```python
from build123d import *

# Parameters (mm, degrees)
SKETCH1_W           = 57.15
SKETCH1_H           = 50.00625
SKETCH1_W_2         = 44.45
SKETCH1_H_2         = 37.30625
BOSS_EXTRUDE1_DEPTH = 12.7
SKETCH2_W           = 57.15
SKETCH2_H           = 50.00625
SKETCH2_R           = 6.35
BOSS_EXTRUDE2_DEPTH = 3.175
SKETCH4_W           = 12.7
SKETCH4_H           = 3.175
BOSS_EXTRUDE3_DEPTH = 12.7
SKETCH5_R           = 2.4892
CUT_EXTRUDE1_DEPTH  = 3.175
FILLET1_R           = 1.27
SKETCH6_R           = 1.5875
CUT_EXTRUDE2_DEPTH  = 9.525


with BuildPart() as part:
    # Sketch1 → Boss-Extrude1 (new body)
    with BuildSketch(Plane.XY):
        Rectangle(SKETCH1_W, SKETCH1_H)
        Rectangle(SKETCH1_W_2, SKETCH1_H_2, mode=Mode.SUBTRACT)
    extrude(amount=BOSS_EXTRUDE1_DEPTH)

    # Sketch2 → Boss-Extrude2 (add)
    with BuildSketch(Plane.XY):
        Rectangle(SKETCH2_W, SKETCH2_H)
        Circle(SKETCH2_R, mode=Mode.SUBTRACT)
    extrude(amount=-BOSS_EXTRUDE2_DEPTH)

    # Sketch4 → Boss-Extrude3 (add)
    with BuildSketch(Plane.XY):
        with Locations((-34.925, -23.415625)):
            Rectangle(SKETCH4_W, SKETCH4_H)
        with Locations((34.925, -23.415625)):
            Rectangle(SKETCH4_W, SKETCH4_H)
    extrude(amount=BOSS_EXTRUDE3_DEPTH)

    # Sketch5 → Cut-Extrude1 (cut)
    with BuildSketch(Plane(origin=(0, -21.828125, 0), x_dir=(1, 0, 0), z_dir=(0, 1, 0))):
        with Locations(Location((-34.925, -6.35, 0), (0, 0, 180))):
            Circle(SKETCH5_R)
        with Locations(Location((34.925, -6.35, 0), (0, 0, 180))):
            Circle(SKETCH5_R)
    extrude(amount=-CUT_EXTRUDE1_DEPTH, mode=Mode.SUBTRACT)

    # Fillet1
    fillet1_edges = [part.edges().sort_by_distance(p)[0] for p in [
        (-22.225, 0, 0),
        (0, -18.653125, 0),
        (22.225, 0, 0),
        (0, 18.653125, 0),
    ]]
    fillet(fillet1_edges, radius=FILLET1_R)

    # Sketch6 → Cut-Extrude2 (cut)
    with BuildSketch(Plane.XY.offset(12.7)):
        with Locations((-25.4, 21.828125)):
            Circle(SKETCH6_R)
        with Locations((25.4, 21.828125)):
            Circle(SKETCH6_R)
        with Locations((25.4, -21.828125)):
            Circle(SKETCH6_R)
        with Locations((-25.4, -21.828125)):
            Circle(SKETCH6_R)
    extrude(amount=-CUT_EXTRUDE2_DEPTH, mode=Mode.SUBTRACT)


solid = part.part
```
For this review, take the finished solid that the model builds, in its own axes (mm). A direction names the side the tool comes from. Round coordinates to 2 decimals unless told otherwise and drop trailing zeros. Write each loop counter-clockwise with the first axis right and the second up, starting at its lowest first coordinate (ties: lowest second). Pieces come first, ordered by that corner, then holes.
1) Insertion check: pin 1 Ø1 at (x, y) = (-25.5, -22.5) entering from +Z (3 decimals); pin 2 Ø1 at (x, y) = (12, 5) entering from +Z; pin 3 Ø1 at (x, y) = (-37.5, -24) entering from -Z; pin 4 Ø4.5 at (x, z) = (-34.925, 6.35) entering from +Y. Each pin has a flat end and moves straight along its axis. Give the tip position at first contact, or say it passes through.
Answer below:
pin 1: stops at z = 3.175
pin 2: stops at z = 0
pin 3: stops at z = 0
pin 4: passes through
2) Take a section at D-D on x = 0. Give the boundary of the cut face in (y, z) (3 decimals).
Answer below:
outline: (-25.003, -3.175) - (-6.35, -3.175) - (-6.35, 0) - (-17.383, 0) arc R1.27 cw to (-18.653, 1.27) - (-18.653, 12.7) - (-25.003, 12.7) - close; (6.35, -3.175) - (25.003, -3.175) - (25.003, 12.7) - (18.653, 12.7) - (18.653, 1.27) arc R1.27 cw to (17.383, 0) - (6.35, 0) - close
3) Mouldability with a two-part tool opening along Z and no side actions: class faces 1 (the face through (32.626, -23.393, 5.397)), 2 (the face through (38, -21.828, 6)), 3 (the face through (-25, 22, 3.175)) as +Z half, -Z half, draft (parallel to the pull), parting line (faces both ways), or undercut.
Answer below:
face 1: undercut
face 2: draft
face 3: +Z half
4) Take a section at B-B on x = -25.4. Give the boundary of the cut face in (y, z) (3 decimals).
Answer below:
outline: (-25.003, -3.175) - (25.003, -3.175) - (25.003, 12.7) - (23.416, 12.7) - (23.416, 3.175) - (20.241, 3.175) - (20.241, 12.7) - (-20.241, 12.7) - (-20.241, 3.175) - (-23.416, 3.175) - (-23.416, 12.7) - (-25.003, 12.7) - close
5) For line 1 along X through (y, z) = (-8.5, 8) (3 decimals); line 2 along X through (y, z) = (20.5, 5) (3 decimals); line 3 along Y through (x, z) = (9.5, 6.75), list the stretches that pass through material, from the lowest coordinate up.
Answer below:
line 1: x = -28.575 to -22.225, 22.225 to 28.575
line 2: x = -28.575 to -26.27, -24.53 to 24.53, 26.27 to 28.575
line 3: y = -25 to -18.65, 18.65 to 25
6) Take a section at A-A on z = 7.25. Give the boundary of the cut face in (x, y) (1 decimal).
Answer below:
outline: (-41.3, -25) - (-37.2, -25) - (-37.2, -21.8) - (-41.3, -21.8) - close; (-32.6, -25) - (32.6, -25) - (32.6, -21.8) - (28.6, -21.8) - (28.6, 25) - (-28.6, 25) - (-28.6, -21.8) - (-32.6, -21.8) - close; (37.2, -25) - (41.3, -25) - (41.3, -21.8) - (37.2, -21.8) - close; hole circle Ø3.2 at (-25.4, -21.8); hole circle Ø3.2 at (-25.4, 21.8); hole (-22.2, -18.7) - (22.2, -18.7) - (22.2, 18.7) - (-22.2, 18.7) - close; hole circle Ø3.2 at (25.4, -21.8); hole circle Ø3.2 at (25.4, 21.8)
7) Take a section at C-C on y = 0. Give the boundary of the cut face in (x, z) (3 decimals).
Answer below:
outline: (-28.575, -3.175) - (-6.35, -3.175) - (-6.35, 0) - (-20.955, 0) arc R1.27 cw to (-22.225, 1.27) - (-22.225, 12.7) - (-28.575, 12.7) - close; (6.35, -3.175) - (28.575, -3.175) - (28.575, 12.7) - (22.225, 12.7) - (22.225, 1.27) arc R1.27 cw to (20.955, 0) - (6.35, 0) - close
8) Machinability: for faces 4 (the face through (35, -23, 0)), 5 (the face through (26.13, 20.42, 8)), 6 (the face through (-7, 0, -3.175)), which of the approach directions +Z, -Z, +X, -X, +Y, -Y give a long, thin tool a straight path to every point of the face, cutting with its end or side? Answer none if there is none.
Answer below:
face 4: -Z, +X, +Y, -Y
face 5: +Z
face 6: -Z, +X, -X, +Y, -Y
